Autodesk Inventor part; units mm, degrees
ref_plane "YZ Plane" through (0, 0, 0) normal (1, 0, 0) x (0, 1, 0)
ref_plane "XZ Plane" through (0, 0, 0) normal (0, 1, 0) x (-1, 0, 0)
ref_plane "XY Plane" through (0, 0, 0) normal (0, 0, 1) x (1, 0, 0)
sketch "Skizze1" plane through (0, 0, 0) normal (0, 0, 1) x (1, 0, 0)
  line L0 (0, 22.4) -> (0, -22.4)
  line L1 (-22.4, 0) -> (22.4, 0)
  line L2 (-16, 16) -> (16, 16)
  line L3 (16, 16) -> (16, -16)
  line L4 (16, -16) -> (-16, -16)
  line L5 (-16, -16) -> (-16, 16)
  circle A0 centre (0, 0) radius 12.1
  dimension "d0" = 32
  dimension "d1" = 32
  dimension "d2" = 24.2
extrude "Extrusion1" add sketch "Skizze1" along normal blind 14 contours L2 L3 L1 A0 L0 | L0 A0 L1 L5 L2 | L1 L3 L4 L0 A0 | A0 L0 L4 L5 L1
sketch "Skizze2" plane through (16, -16, 0) normal (1, 0, 0) x (0, 0, -1)
  line L0 (-14, 32) -> (-14, 0)
  line L1 (0, 32) -> (0, 0)
  line L2 (-14, 0) -> (0, 0)
  line L3 (0, 0) -> (0, 3)
  line L4 (0, 3) -> (-14, 3)
  line L5 (-14, 3) -> (-14, 0)
  point P0 (0, 16)
  point P1 (-14, 3)
  dimension "d5" = 3
sketch "Skizze3" plane through (-16, -16, 0) normal (-1, 0, 0) x (0, 0, 1)
  line L0 (14, 32) -> (14, 0)
  line L1 (0, 32) -> (0, 0)
  line L2 (14, 0) -> (0, 0)
  line L3 (0, 0) -> (0, 3)
  line L4 (0, 3) -> (14, 3)
  line L5 (14, 3) -> (14, 0)
  point P0 (0, 16)
  point P1 (14, 3)
  dimension "d6" = 3
extrude "Extrusion2" add sketch "Skizze3" along normal blind 10.5
extrude "Extrusion3" add sketch "Skizze2" along normal blind 10.5
sketch "Skizze4" plane through (0, 0, 0) normal (0, 0, -1) x (-1, 0, 0)
  circle A0 centre (0, 0) radius 12.1
  circle A1 centre (0, 0) radius 12.1
  circle A2 centre (0, 0) radius 9
  dimension "d11" = 24.2
  dimension "d12" = 18
extrude "Extrusion4" add sketch "Skizze4" against normal blind 9
fillet "Rundung1" radius 16 2 edges at (16, 16, 7) (-16, 16, 7)
sketch "Skizze5" plane through (16, -13, 14) normal (0, 1, 0) x (1, 0, 0)
  circle A0 centre (-39, 10.5) radius 1.6
  line L0 (-32, 14) -> (-42.5, 14)
  line L1 (-42.5, 0) -> (-42.5, 14)
  circle A1 centre (7, 10.5) radius 1.6
  line L2 (0, 14) -> (10.5, 14)
  line L3 (10.5, 14) -> (10.5, 0)
  point P0 (-16, 14)
  dimension "d16" = 3.2
  dimension "d17" = 3.5
  dimension "d18" = 3.5
  dimension "d19" = 3.2
  dimension "d20" = 3.5
  dimension "d21" = 3.5
extrude "Extrusion5" cut sketch "Skizze5" against normal up to surface (3 mm away)
fillet "Rundung2" radius 1 2 edges at (-16, -13, 7) (16, -13, 7)
sketch "Skizze6" plane through (-26.5, -16, 0) normal (0, -1, 0) x (1, 0, 0)
  line L0 (53, 14) -> (0, 14)
  line L1 (53, 14) -> (53, 0)
  line L2 (0, 14) -> (53, 14)
  line L3 (53, 14) -> (53, 0)
  line L4 (53, 0) -> (0, 0)
  line L5 (0, 0) -> (0, 14)
  circle A0 centre (3.5, 3.5) radius 1.6
  circle A1 centre (3.5, 3.5) radius 1.6
  circle A2 centre (49.5, 3.5) radius 1.6
  circle A3 centre (49.5, 3.5) radius 1.6
  point P0 (26.5, 0)
  dimension "d25" = 3.2
  dimension "d26" = 3.2
extrude "Extrusion6" add sketch "Skizze6" along normal blind 1.5
properties part number "_3D-Druck"
For this review, take the finished solid that the model builds, in its own axes (mm). A direction names the side the tool comes from. Give positions to 0.01 mm unless a question says otherwise; leave off trailing zeros. Order: outer loops, then holes, each group sorted by start corner. A loop starts at its lowest first (then second) coordinate and runs counter-clockwise, first axis right, second up. Notation, with made-up numbers: (-24.75, 71) - (29.25, 71) arc R8 cw to (29.25, 78) - close; hole circle Ø8 at (74, 24). An arc over 180 degrees is marked (long way). Answer as a JSON object with one key per item and string values. Group by question number.
Item 1: Machinability: for faces 1 (the flat face through (22, -13, 7)), 2 (the flat face through (2, 9, 9)), 3 (the flat face through (-22, -13, 7)), which of the approach directions +Z, -Z, +X, -X, +Y, -Y give a long, thin tool a straight path to every point of the face, cutting with its end or side? Answer none if there is none.
Item 2: Wall thickness on line 1 along X through (y, z) = (-16.6, 3.5); line 2 along Y through (x, z) = (0, 2); line 3 along Y through (x, z) = (0, 10.9): over which ranges is each line inside the solid? List them lowest first.
Item 3: Take a section at B-B on x = 23. Give the boundary of the cut face in (y, z).
Item 4: Draft analysis for pull direction Y (two halves, no side actions). For faces 4 (the cylindrical face through (-16.301, -12.715, 7.098)), 5 (the cylindrical face through (11.18, 4.63, 11.46)), 6 (the flat face through (-26.5, -15, 7)), state which applies: pulls with the +Y half, pulls with the -Y half, needs draft (parallel to the pull), parting line crosses it, or undercut.
Item 5: Take a section at A-A on z = 3.5. Give the number of separate pieces and of enclosed holes in the cut face, and give its area (3 significant figures).
Item 6: Take a section at C-C on y = -3. Give the boundary of the cut face in (x, z).
Item 7: Clearance check with flat-ended pins moving along their axes: pin 1 Ø6 at (x, y) = (21, 2.5) entering from +Z; pin 2 Ø2 at (x, y) = (-9, -1) entering from +Z; pin 3 Ø3 at (x, z) = (-4.5, 6) entering from +Y; pin 4 Ø4 at (y, z) = (7, 11.5) entering from -X. State where each tip first meets the part, or that it passes through.
Reported:
{
 "1": {"face 1": "+Z, -Z, +X, +Y", "face 2": "+Z", "face 3": "+Z, -Z, -X, +Y"},
 "2": {"line 1": "-26.5 to -24.6, -21.4 to 21.4, 24.6 to 26.5", "line 2": "-17.5 to -9, 9 to 16", "line 3": "-17.5 to -12.1, 12.1 to 16"},
 "3": {"outline": "(-17.5, 0) - (-13, 0) - (-13, 1.9) - (-17.5, 1.9) - close; (-17.5, 5.1) - (-13, 5.1) - (-13, 14) - (-17.5, 14) - close"},
 "4": {"face 4": "pulls with the +Y half", "face 5": "undercut", "face 6": "needs draft"},
 "5": {"separate pieces": "3", "enclosed holes": "1", "area": "774 mm^2"},
 "6": {"outline": "(-16, 0) - (-8.49, 0) - (-8.49, 9) - (-11.72, 9) - (-11.72, 14) - (-16, 14) - close; (8.49, 0) - (16, 0) - (16, 14) - (11.72, 14) - (11.72, 9) - (8.49, 9) - close"},
 "7": {"pin 1": "through", "pin 2": "z = 9", "pin 3": "y = 15.72", "pin 4": "x = -15.2"}
}
